Geometry check sheet. Reference: the model listing, model coordinates, mm. A direction names the side the tool comes from. Round coordinates to 2 decimals unless told otherwise and drop trailing zeros. Order: outer loops, then holes, each group sorted by start corner. A loop starts at its lowest first (then second) coordinate and runs counter-clockwise, first axis right, second up. Notation, with made-up numbers: (26, 36.5) - (66, 36.5) arc R18 ccw to (66, 69.5) - close; hole circle Ø10 at (-23.75, 8). An arc over 180 degrees is marked (long way). One line per question, with ' | ' between items. Start each with the question number.
Q1. Sectioned sample at B-B, the plane y = 6.5. Enter the section's corners in (x, z).
Q2. Tool access check on faces 4 (the face through (29.715, 11.699, 0.247)), 5 (the face through (28, 5.9, 0.5)). Record the directions out of +Z, -Z, +X, -X, +Y, -Y that give a thin tool (end or side, any length) a straight path to the whole face; none if there is none.
Q3. Sectioned sample at A-A, the plane x = 11. Enter the section's corners in (y, z), then the cut area to 3 significant figures.
Q4. Sectioned sample at C-C, the plane z = 1.25. Enter the section's corners in (x, y), then the cut area to 3 significant figures.
Q5. Mould release check, pull along X, two halves, no side actions. Record for faces 1 (the face through (0.285, 5.93, 1.199)), 2 (the face through (14.9, 11.8, 0)), 3 (the face through (14.8, 11.5, 0.5)): +X half, -X half, draft (parallel to the pull), parting line (faces both ways), or undercut.
Q6. Gauge pin test, flat end, axial feed: P1, Ø5.5, axis at x = 13.5, y = 3.5, coming from the -Z side. Record the tip position at first contact, or that the pin passes through.
Q7. Material ranges on line 1 along X through (y, z) = (1, 0.4); line 2 along Y through (x, z) = (3, 0.3); line 3 along Z through (x, y) = (6.5, 7.25), recorded low to high.
```python
from build123d import *

# Parameters (mm, degrees)
F1_DEPTH = 1.5
F2_R     = 1
F3_W     = 26
F3_H     = 11
F4_DEPTH = 1


with BuildPart() as f1:
    # F0 (on Top) → F1 (new body)
    with BuildSketch(Plane.XY):
        with BuildLine():
            ThreePointArc((0, 1), (0.2928932188, 0.2928932188), (1, 0))
            Line((1, 0), (29, 0))
            ThreePointArc((29, 0), (29.7071067812, 0.2928932188), (30, 1))
            Line((30, 1), (30, 11))
            ThreePointArc((30, 11), (29.7071067812, 11.7071067812), (29, 12))
            Line((29, 12), (1, 12))
            ThreePointArc((1, 12), (0.2928932188, 11.7071067812), (0, 11))
            Line((0, 11), (0, 1))
        make_face()
    extrude(amount=F1_DEPTH)

    # F2
    f2_edges = [f1.edges().sort_by_distance(p)[0] for p in [
        (0, 6, 1.5),
        (0.292893, 0.292893, 1.5),
        (15, 0, 1.5),
        (29.707107, 0.292893, 1.5),
        (30, 6, 1.5),
        (29.707107, 11.707107, 1.5),
        (15, 12, 1.5),
        (0.292893, 11.707107, 1.5),
    ]]
    fillet(f2_edges, radius=F2_R)

    # F3 (on Top) → F4 (cut)
    with BuildSketch(Plane.XY):
        with Locations((15, 6)):
            Rectangle(F3_W, F3_H)
    extrude(amount=F4_DEPTH, mode=Mode.SUBTRACT)


solid = f1.part
```
Determined:
1) outline: (0, 0) - (2, 0) - (2, 1) - (28, 1) - (28, 0) - (30, 0) - (30, 0.5) arc R1 ccw to (29, 1.5) - (1, 1.5) arc R1 ccw to (0, 0.5) - close
2) face 4: +Z, -Z, +X, +Y | face 5: -Z
3) outline: (0, 0) - (0.5, 0) - (0.5, 1) - (11.5, 1) - (11.5, 0) - (12, 0) - (12, 0.5) arc R1 ccw to (11, 1.5) - (1, 1.5) arc R1 ccw to (0, 0.5) - close | area: 6.57 mm2
4) outline: (0.34, 1) arc R0.66 ccw to (1, 0.34) - (29, 0.34) arc R0.66 ccw to (29.66, 1) - (29.66, 11) arc R0.66 ccw to (29, 11.66) - (1, 11.66) arc R0.66 ccw to (0.34, 11) - close | area: 332 mm2
5) face 1: -X half | face 2: draft | face 3: undercut
6) P1: stops at z = 1
7) line 1: x = 0 to 2, 28 to 30 | line 2: y = 0 to 0.5, 11.5 to 12 | line 3: z = 1 to 1.5
